```python
from build123d import *

# Parameters (mm, degrees)
CROQUIS1_W              = 20
CROQUIS1_H              = 20
CROQUIS1_R              = 3
SALIENTE_EXTRUIR1_DEPTH = 5
SALIENTE_EXTRUIR2_DEPTH = 2
SALIENTE_EXTRUIR3_DEPTH = 8
SALIENTE_EXTRUIR4_DEPTH = 1.2
CROQUIS5_W              = 10
CROQUIS5_H              = 92
SALIENTE_EXTRUIR5_DEPTH = 2
CROQUIS6_W              = 83
CROQUIS6_H              = 62
CORTAR_EXTRUIR1_DEPTH   = 6


with BuildPart() as part:
    # Croquis1 → Saliente-Extruir1 (new body)
    with BuildSketch(Plane(origin=(0, 0, 0), x_dir=(1, 0, 0), z_dir=(0, 1, 0))):
        Rectangle(CROQUIS1_W, CROQUIS1_H)
        Circle(CROQUIS1_R, mode=Mode.SUBTRACT)
        with BuildLine():
            Line((2.321637353, -1.9), (-2.321637353, -1.9))
            ThreePointArc((-2.321637353, -1.9), (0, -3), (2.321637353, -1.9))
        make_face()
        with BuildLine():
            Line((-2.321637353, 1.9), (2.321637353, 1.9))
            ThreePointArc((2.321637353, 1.9), (0, 3), (-2.321637353, 1.9))
        make_face()
    extrude(amount=SALIENTE_EXTRUIR1_DEPTH)

    # Croquis2 → Saliente-Extruir2 (add)
    with BuildSketch(Plane(origin=(0, 5, 0), x_dir=(1, 0, 0), z_dir=(0, 1, 0))):
        Polygon((-10, 10), (-39.5, 10), (-39.5, 0), (-39.5, -80), (39.5, -80), (39.5, 0), (39.5, 10), (10, 10), align=None)
    extrude(amount=SALIENTE_EXTRUIR2_DEPTH)

    # Croquis3 → Saliente-Extruir3 (add)
    with BuildSketch(Plane.XZ.offset(-5)):
        Polygon((39.5, 80), (39.5, -10), (41.5, -10), (41.5, 82), (-41.5, 82), (-41.5, -10), (-39.5, -10), (-39.5, 80), align=None)
    extrude(amount=-SALIENTE_EXTRUIR3_DEPTH)

    # Croquis4 → Saliente-Extruir4 (add)
    with BuildSketch(Plane(origin=(0, 13, 0), x_dir=(1, 0, 0), z_dir=(0, 1, 0))):
        Polygon((-39.5, -80), (-29.5, -80), (-39.5, -70), align=None)
        Polygon((-29.5, -82), (-29.5, -80), (-39.5, -80), (-39.5, -70), (-41.5, -70), (-41.5, -82), align=None)
        Polygon((39.5, -70), (29.5, -80), (39.5, -80), align=None)
        Polygon((39.5, -80), (29.5, -80), (29.5, -82), (41.5, -82), (41.5, -70), (39.5, -70), align=None)
    extrude(amount=SALIENTE_EXTRUIR4_DEPTH)

    # Croquis5 → Saliente-Extruir5 (add)
    with BuildSketch(Plane.XZ.offset(-5)):
        with Locations((-46.5, 36)):
            Rectangle(CROQUIS5_W, CROQUIS5_H)
        with BuildLine():
            Line((-48.5, 0), (-48.5, 72))
            ThreePointArc((-48.5, 72), (-46.5, 74), (-44.5, 72))
            Line((-44.5, 72), (-44.5, 0))
            ThreePointArc((-44.5, 0), (-46.5, -2), (-48.5, 0))
        make_face(mode=Mode.SUBTRACT)
        with Locations((46.5, 36)):
            Rectangle(CROQUIS5_W, CROQUIS5_H)
        with BuildLine():
            Line((48.5, 0), (48.5, 72))
            ThreePointArc((48.5, 72), (46.5, 74), (44.5, 72))
            Line((44.5, 72), (44.5, 0))
            ThreePointArc((44.5, 0), (46.5, -2), (48.5, 0))
        make_face(mode=Mode.SUBTRACT)
    extrude(amount=-SALIENTE_EXTRUIR5_DEPTH)

    # Croquis6 → Cortar-Extruir1 (cut)
    with BuildSketch(Plane(origin=(0, 13, 0), x_dir=(1, 0, 0), z_dir=(0, 1, 0))):
        with Locations((0, -21)):
            Rectangle(CROQUIS6_W, CROQUIS6_H)
    extrude(amount=-CORTAR_EXTRUIR1_DEPTH, mode=Mode.SUBTRACT)


solid = part.part
```
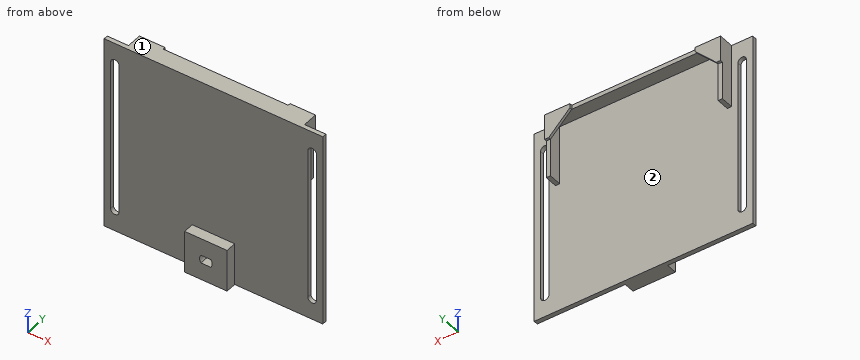
The listing builds one solid part. Answer for the finished solid, in the listing's coordinates (mm). Face numbers are marked on the shaded views. Give positions to 0.01 mm unless a question says otherwise; leave off trailing zeros. Order: outer loops, then holes, each group sorted by start corner. A loop starts at its lowest first (then second) coordinate and runs counter-clockwise, first axis right, second up.
Item 1: The part is cut by section A-A, the plane z = 35. Give the vertices of the cut face in (x, y).
From the geometry:
outline: (-51.5, 5) - (-48.5, 5) - (-48.5, 7) - (-51.5, 7) - close; (-44.5, 5) - (44.5, 5) - (44.5, 7) - (-44.5, 7) - close; (48.5, 5) - (51.5, 5) - (51.5, 7) - (48.5, 7) - close
Item 2: Given pin 1 Ø12 at (x, z) = (-20, 16.5) entering from +Y; pin 2 Ø1.3 at (y, z) = (13.5, 81) entering from +X; pin 3 Ø5.5 at (y, z) = (1.5, 3.5) entering from +X, each flat-ended and moving along its own axis, determine where each tip first touches the part or whether it passes through.
From the geometry:
pin 1: stops at y = 7
pin 2: stops at x = 41.5
pin 3: stops at x = 10
Item 3: The part is cut by section B-B, the plane x = 46.5. Give the vertices of the cut face in (y, z), and give its area (3 significant figures).
From the geometry:
outline: (5, -10) - (7, -10) - (7, -2) - (5, -2) - close; (5, 74) - (7, 74) - (7, 82) - (5, 82) - close
area: 32.0 mm2
Item 4: Find the intervals of material crossed by probe 1 along X at (y, z) = (5.75, 40.5); probe 2 along X at (y, z) = (10, 65.5); probe 3 along Z at (x, y) = (1.5, 3.5), in increasing order.
From the geometry:
probe 1: x = -51.5 to -48.5, -44.5 to 44.5, 48.5 to 51.5
probe 2: x = -41.5 to -39.5, 39.5 to 41.5
probe 3: z = -10 to -1.9, 1.9 to 10
Item 5: The part is cut by section D-D, the plane x = -34. Give the vertices of the cut face in (y, z).
From the geometry:
outline: (5, -10) - (7, -10) - (7, 80) - (13, 80) - (13, 75.5) - (14.2, 75.5) - (14.2, 82) - (5, 82) - close
Item 6: The part is cut by section C-C, the plane y = 2.25. Give the vertices of the cut face in (x, z), and give its area (3 significant figures).
From the geometry:
outline: (-10, -10) - (10, -10) - (10, 10) - (-10, 10) - close; hole (-2.32, -1.9) - (2.32, -1.9) arc R3 ccw to (2.32, 1.9) - (-2.32, 1.9) arc R3 ccw to start
area: 379 mm2
Item 7: For a pull along X with two mould halves and no side action, classify the marked faces 1 and 2 as pulls with the +X half, pulls with the -X half, needs draft (parallel to the pull), parting line crosses it, or undercut.
From the geometry:
face 1: needs draft
face 2: undercut
